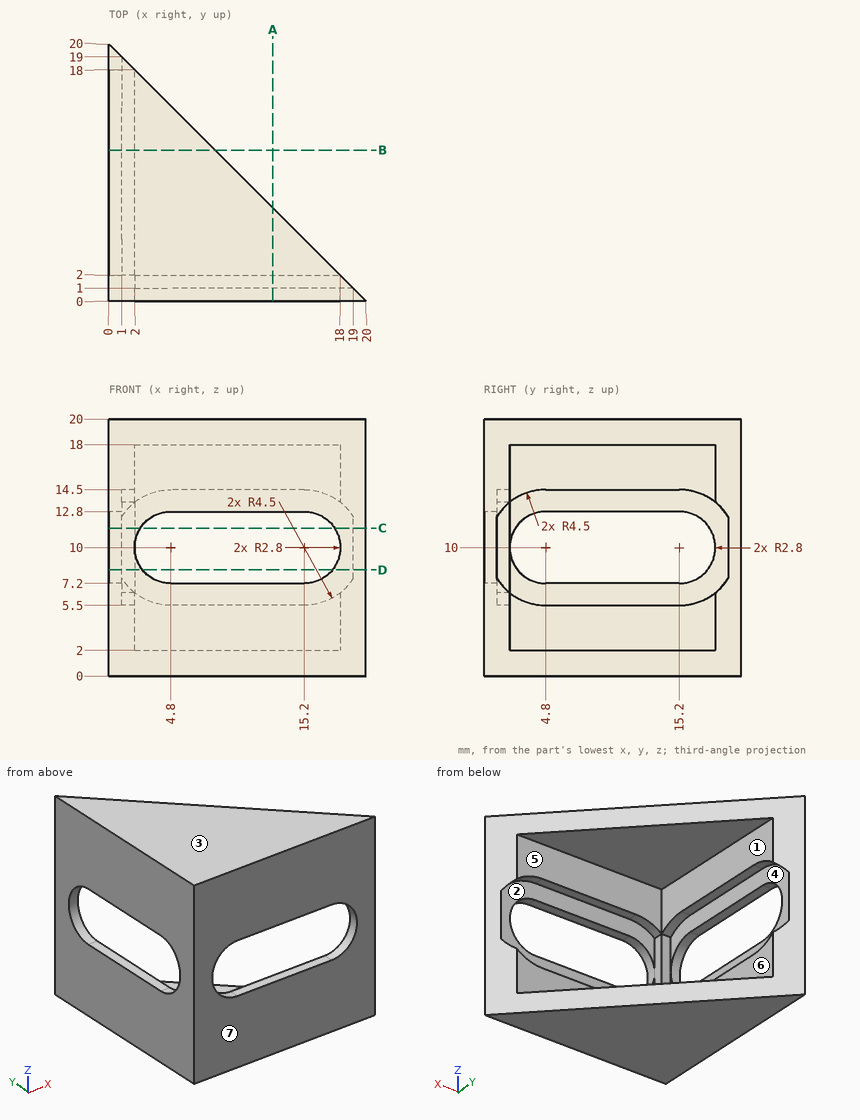
Drawing for the job (mm, zero at the part's lowest x, y, z). A direction names the side the tool comes from. Give positions to 0.01 mm unless a question says otherwise; leave off trailing zeros. Loops run counter-clockwise (first coordinate to the right, second up) from the corner with the lowest first, then second, coordinate; pieces in that order, holes last. Notation, with made-up numbers: M -22.5,8 L 17.5,8 A27 cw 17.5,37 Z; hole C 64.5,27 d4. An arc over 180 degrees is marked long. Use one line per item in the form item = value.
Item 1: Drill centre lines: probe 1 along Z at (x, y) = (12.5, 1.5); probe 2 along Z at (x, y) = (10, 8.25); probe 3 along Y at (x, z) = (11, 2.5). Where is each one in solid material? Low to high. Write a range as from..to.
Determined:
probe_1 = 0..5.5, 14.5..20
probe_2 = 0..2, 18..20
probe_3 = 0..2
Item 2: Slice it at A-A (x = 12.75). List the corners of the cut face in (y, z), plus the area to 3 significant figures.
Determined:
outline = M 0,0 L 7.25,0 L 7.25,2 L 2,2 L 2,5.5 L 1,5.5 L 1,7.2 L 0,7.2 Z; M 0,12.8 L 1,12.8 L 1,14.5 L 2,14.5 L 2,18 L 7.25,18 L 7.25,20 L 0,20 Z
area = 46.4 mm2
Item 3: Flat gauge pins, fed straight in: pin 1 (3.5 mm diameter, centred on y = 12, z = 16.5, fed in from +X); pin 2 (5 mm diameter, centred on x = 2.5, y = 11.5, fed in from -Z); pin 3 (8 mm diameter, centred on x = 17.5, z = 8.5, fed in from +Y); pin 4 (2.5 mm diameter, centred on y = 8.5, z = 10.5, fed in from +X). Where does each tip first touch, or does it go through?
Determined:
pin_1 = 8.9
pin_2 = 0
pin_3 = 2
pin_4 = through
Item 4: Which spindle directions (+Z, -Z, +X, -X, +Y, -Y) get a long thin tool onto all of the face, cutting with end or side? Do the marked faces 1, 2 and 3. Say none if no direction does.
Determined:
face_1 = +X, +Y
face_2 = +Y
face_3 = +Z, +X, -X, +Y, -Y
Item 5: Slice it at C-C (z = 11.5). List the corners of the cut face in (x, y).
Determined:
outline = M 0,0 L 2.44,0 L 2.44,1 L 2,1 L 2,2 L 1,2 L 1,2.44 L 0,2.44 Z; M 0,17.56 L 1,17.56 L 1,19 L 0,20 Z; M 17.56,0 L 20,0 L 19,1 L 17.56,1 Z
Item 6: Two-plate mould, pull along Y, no slides. Class the marked faces 4, 5, 6 and 7: pulls with the +Y half, pulls with the -Y half, needs draft (parallel to the pull), parting line crosses it, or undercut.
Determined:
face_4 = undercut
face_5 = pulls with the +Y half
face_6 = needs draft
face_7 = pulls with the -Y half
Item 7: Slice it at B-B (y = 11.75). List the corners of the cut face in (x, z), plus the area to 3 significant figures.
Determined:
outline = M 0,0 L 8.25,0 L 8.25,2 L 2,2 L 2,5.5 L 1,5.5 L 1,7.2 L 0,7.2 Z; M 0,12.8 L 1,12.8 L 1,14.5 L 2,14.5 L 2,18 L 8.25,18 L 8.25,20 L 0,20 Z
area = 50.4 mm2
Item 8: Slice it at D-D (z = 8.25). List the corners of the cut face in (x, y), plus the area to 3 significant figures.
Determined:
outline = M 0,0 L 2.61,0 L 2.61,1 L 2,1 L 2,2 L 1,2 L 1,2.61 L 0,2.61 Z; M 0,17.39 L 1,17.39 L 1,19 L 0,20 Z; M 17.39,0 L 20,0 L 19,1 L 17.39,1 Z
area = 9.46 mm2
